```python
from build123d import *

# Parameters (mm, degrees)
SM_BASE_FLANGE_1_DEPTH = 394
SKETCH_6_W             = 30
SKETCH_6_H             = 60
CUT_EXTRUDE_1_DEPTH    = 24
CUT_EXTRUDE_START      = -22
SKETCH_11_W            = 4
SKETCH_11_H            = 77
CUT_EXTRUDE_6_DEPTH    = 22
SKETCH_8_R             = 8.25
SKETCH_8_R_2           = 3.25
CUT_EXTRUDE_3_DEPTH    = 10
SKETCH_12_R            = 2.5
CUT_EXTRUDE_7_DEPTH    = 10
SKETCH_13_R            = 5
CUT_EXTRUDE_8_DEPTH    = 10
SKETCH_14_R            = 4.5
CUT_EXTRUDE_9_DEPTH    = 10
SKETCH_15_R            = 3.5
CUT_EXTRUDE_10_DEPTH   = 10


# Sheet-metal steps are written as plain solids
with BuildPart() as part:
    # Sketch 1 → Базовая кромка1 (new, symmetric)
    with BuildSketch(Plane.XY):
        with BuildLine():
            Line((0, 0), (0, -18))
            ThreePointArc((0, -18), (-1.171572875, -20.828427125), (-4, -22))
            Line((-4, -22), (-26, -22))
            ThreePointArc((-26, -22), (-27.414213562, -22.585786438), (-28, -24))
            Line((-28, -24), (-28, -116))
            ThreePointArc((-28, -116), (-27.414213562, -117.414213562), (-26, -118))
            Line((-26, -118), (5, -118))
            Line((5, -118), (5, -120))
            Line((5, -120), (-26, -120))
            ThreePointArc((-26, -120), (-28.828427125, -118.828427125), (-30, -116))
            Line((-30, -116), (-30, -24))
            ThreePointArc((-30, -24), (-28.828427125, -21.171572875), (-26, -20))
            Line((-26, -20), (-4, -20))
            ThreePointArc((-4, -20), (-2.585786438, -19.414213562), (-2, -18))
            Line((-2, -18), (-2, 0))
            Line((-2, 0), (0, 0))
        make_face()
    extrude(amount=SM_BASE_FLANGE_1_DEPTH, both=True)

    # Эскиз6 → Вырез-Вытянуть1 (cut)
    with BuildSketch(Plane(origin=(0, 0, 0), x_dir=(1, 0, 0), z_dir=(0, 1, 0))):
        with Locations((-15, -364)):
            Rectangle(SKETCH_6_W, SKETCH_6_H)
        with Locations((-15, 364)):
            Rectangle(SKETCH_6_W, SKETCH_6_H)
    extrude(amount=-CUT_EXTRUDE_1_DEPTH, mode=Mode.SUBTRACT)

    # Эскиз11 → Вырез-Вытянуть6 (cut)
    with BuildSketch(Plane(origin=(0, 0, 0), x_dir=(1, 0, 0), z_dir=(0, 1, 0)).offset(CUT_EXTRUDE_START)):
        with Locations((-2, 295.5)):
            Rectangle(SKETCH_11_W, SKETCH_11_H)
        with Locations((-2, -295.5)):
            Rectangle(SKETCH_11_W, SKETCH_11_H)
    extrude(amount=CUT_EXTRUDE_6_DEPTH, mode=Mode.SUBTRACT)

    # Эскиз8 → Вырез-Вытянуть3 (cut)
    with BuildSketch(Plane.ZY.offset(30)):
        with Locations(Location((-365, -70, 0), (0, 0, 270))):
            Circle(SKETCH_8_R)
        with Locations(Location((-325, -70, 0), (0, 0, 270))):
            Circle(SKETCH_8_R)
        with Locations(Location((-365, -50, 0), (0, 0, 270))):
            Circle(SKETCH_8_R_2)
        with Locations(Location((-365, -100, 0), (0, 0, 270))):
            Circle(SKETCH_8_R_2)
        with Locations(Location((-285, -50, 0), (0, 0, 270))):
            Circle(SKETCH_8_R_2)
        with Locations(Location((-285, -100, 0), (0, 0, 270))):
            Circle(SKETCH_8_R_2)
        with Locations(Location((285, -100, 0), (0, 0, 90))):
            Circle(SKETCH_8_R_2)
        with Locations(Location((285, -50, 0), (0, 0, 90))):
            Circle(SKETCH_8_R_2)
        with Locations(Location((365, -100, 0), (0, 0, 90))):
            Circle(SKETCH_8_R_2)
        with Locations(Location((365, -50, 0), (0, 0, 90))):
            Circle(SKETCH_8_R_2)
        with Locations(Location((325, -70, 0), (0, 0, 90))):
            Circle(SKETCH_8_R)
        with Locations(Location((365, -70, 0), (0, 0, 90))):
            Circle(SKETCH_8_R)
    extrude(amount=-CUT_EXTRUDE_3_DEPTH, mode=Mode.SUBTRACT)

    # Эскиз12 → Вырез-Вытянуть7 (cut)
    with BuildSketch(Plane.ZY.offset(2)):
        with Locations(Location((-237, -7, 0), (0, 0, 270))):
            Circle(SKETCH_12_R)
        with Locations(Location((-227, -7, 0), (0, 0, 270))):
            Circle(SKETCH_12_R)
        with Locations(Location((227, -7, 0), (0, 0, 90))):
            Circle(SKETCH_12_R)
        with Locations(Location((237, -7, 0), (0, 0, 90))):
            Circle(SKETCH_12_R)
    extrude(amount=-CUT_EXTRUDE_7_DEPTH, mode=Mode.SUBTRACT)

    # Эскиз13 → Вырез-Вытянуть8 (cut)
    with BuildSketch(Plane(origin=(0, -20, 0), x_dir=(1, 0, 0), z_dir=(0, 1, 0))):
        with Locations(Location((-14, 300, 0), (0, 0, 180))):
            Circle(SKETCH_13_R)
        with Locations((-14, -300)):
            Circle(SKETCH_13_R)
    extrude(amount=-CUT_EXTRUDE_8_DEPTH, mode=Mode.SUBTRACT)

    # Эскиз14 → Вырез-Вытянуть9 (cut)
    with BuildSketch(Plane(origin=(0, -118, 0), x_dir=(1, 0, 0), z_dir=(0, 1, 0))):
        with Locations(Location((-10, 230, 0), (0, 0, 180))):
            Circle(SKETCH_14_R)
        with Locations((-10, -230)):
            Circle(SKETCH_14_R)
    extrude(amount=-CUT_EXTRUDE_9_DEPTH, mode=Mode.SUBTRACT)

    # Эскиз15 → Вырез-Вытянуть10 (cut)
    with BuildSketch(Plane(origin=(0, 0, 0), x_dir=(0, 0, -1), z_dir=(1, 0, 0))):
        with Locations(Location((-200, -7, 0), (0, 0, 90))):
            Circle(SKETCH_15_R)
        with Locations(Location((200, -7, 0), (0, 0, 270))):
            Circle(SKETCH_15_R)
    extrude(amount=-CUT_EXTRUDE_10_DEPTH, mode=Mode.SUBTRACT)


solid = part.part
```
Geometry: final body of the model. Coordinates: model frame, mm. A direction names the side the tool comes from. Round coordinates to 2 decimals unless told otherwise and drop trailing zeros. Loops run counter-clockwise (first coordinate to the right, second up) from the corner with the lowest first, then second, coordinate; pieces in that order, holes last. Notation, with made-up numbers: (44.25, 69.5) -> (76.25, 69.5) arc R31 ccw to (76.25, 93.5) -> close; hole circle Ø5 at (72.5, 31). An arc over 180 degrees is marked (long way). Use one line per item in the form item = value.
Item 1: Material intervals for probe 1 along Z at (x, y) = (-10, -118.85); probe 2 along Z at (x, y) = (-28.6, -50); probe 3 along Y at (x, z) = (-12.5, 307.5), sorted ascending.
Evaluation:
probe_1 = -394 to -234.5, -225.5 to 225.5, 234.5 to 394
probe_2 = -394 to -368.25, -361.75 to -288.25, -281.75 to 281.75, 288.25 to 361.75, 368.25 to 394
probe_3 = -120 to -118, -22 to -20
Item 2: Access query for faces 5 (the flat face through (-2, -9, 4)), 6 (the flat face through (-10, -120, 6)), 7 (the flat face through (0, -9, 4)), 8 (the flat face through (-28, -69, 6)). Directions: +Z, -Z, +X, -X, +Y, -Y. A direction counts if a zero-diameter tool reaches every point of the face in a straight line with its end or side. Return the directions, or none.
Evaluation:
face_5 = +Z, -Z, -X, +Y
face_6 = +Z, -Z, +X, -X, -Y
face_7 = +Z, -Z, +X, +Y
face_8 = +Z, -Z, +X
Item 3: Contact query for flat-ended pins moving along their axis: pin 1 Ø4 at (x, z) = (-6, -175.5) entering from +Y; pin 2 Ø2 at (y, z) = (-98.5, -166.5) entering from +X; pin 3 Ø6.5 at (y, z) = (-7, -227) entering from -X. Output: stop coordinate, or through.
Evaluation:
pin_1 = -20
pin_2 = -28
pin_3 = -2
Item 4: Cut plane B-B on z = 63. Output: boundary loops of the cut face in (x, y).
Evaluation:
outline = (-30, -116) arc R4 ccw to (-26, -120) -> (5, -120) -> (5, -118) -> (-26, -118) arc R2 cw to (-28, -116) -> (-28, -24) arc R2 cw to (-26, -22) -> (-4, -22) arc R4 ccw to (0, -18) -> (0, 0) -> (-2, 0) -> (-2, -18) arc R2 cw to (-4, -20) -> (-26, -20) arc R4 ccw to (-30, -24) -> close
Item 5: Cut plane C-C on y = -36. Output: boundary loops of the cut face in (x, z), then the cut area to 3 significant figures.
Evaluation:
outline = (-30, -394) -> (-28, -394) -> (-28, 394) -> (-30, 394) -> close
area = 1,580 mm2
Item 6: Cut plane A-A on z = 325. Output: boundary loops of the cut face in (x, y).
Evaluation:
outline = (-30, -116) arc R4 ccw to (-26, -120) -> (5, -120) -> (5, -118) -> (-26, -118) arc R2 cw to (-28, -116) -> (-28, -78.25) -> (-30, -78.25) -> close; (-30, -61.75) -> (-28, -61.75) -> (-28, -24) arc R2 cw to (-26, -22) -> (-4, -22) -> (-4, -20) -> (-26, -20) arc R4 ccw to (-30, -24) -> close
Item 7: Draft query along Z for faces 1 (the cylindrical face through (-29.014, -71.788, 373.054)), 2 (the flat face through (-15, -22, 5)), 3 (the flat face through (-29, -75, -394)), 4 (the cylindrical face through (-29.014, -71.788, 333.054)). Return one class per face: released by +Z, released by -Z, zero draft, split by the parting line, or undercut.
Evaluation:
face_1 = undercut
face_2 = zero draft
face_3 = released by -Z
face_4 = undercut
